from build123d import *

# Parameters (mm, degrees)
SALIENTE_EXTRUIR2_DEPTH = 3
CROQUIS2_R              = 1.25
CORTAR_EXTRUIR4_DEPTH   = 5
SALIENTE_EXTRUIR5_START = 9
CROQUIS6_R              = 2
CROQUIS6_R_2            = 1.25
SALIENTE_EXTRUIR5_DEPTH = 9
CROQUIS4_R              = 2
CROQUIS4_R_2            = 1.25
SALIENTE_EXTRUIR4_DEPTH = 5
CORTAR_EXTRUIR5_DEPTH   = 7
REDONDEO1_R             = 2


with BuildPart() as part:
    # Croquis1 → Saliente-Extruir2 (new body)
    with BuildSketch(Plane.XY):
        with BuildLine():
            Line((21.769230769, 25.846153846), (-36.230769231, 25.846153846))
            ThreePointArc((-36.230769231, 25.846153846), (-38.352089574, 24.96747419), (-39.230769231, 22.846153846))
            Line((-39.230769231, 22.846153846), (-39.230769231, -26.153846154))
            ThreePointArc((-39.230769231, -26.153846154), (-38.352089574, -28.275166497), (-36.230769231, -29.153846154))
            Line((-36.230769231, -29.153846154), (21.769230769, -29.153846154))
            ThreePointArc((21.769230769, -29.153846154), (23.890551113, -28.275166497), (24.769230769, -26.153846154))
            Line((24.769230769, -26.153846154), (24.769230769, 22.846153846))
            ThreePointArc((24.769230769, 22.846153846), (23.890551113, 24.96747419), (21.769230769, 25.846153846))
        make_face()
    extrude(amount=SALIENTE_EXTRUIR2_DEPTH)

    # Croquis2 → Cortar-Extruir4 (cut)
    with BuildSketch(Plane(origin=(0, 0, 0), x_dir=(-1, 0, 0), z_dir=(0, 0, -1))):
        with Locations((-21.769230769, 22.846153846)):
            Circle(CROQUIS2_R)
        with Locations((36.230769231, 22.846153846)):
            Circle(CROQUIS2_R)
        with Locations((36.230769231, -26.153846154)):
            Circle(CROQUIS2_R)
        with Locations((-21.769230769, -26.153846154)):
            Circle(CROQUIS2_R)
    extrude(amount=-CORTAR_EXTRUIR4_DEPTH, mode=Mode.SUBTRACT)

    # Croquis6 → Saliente-Extruir5 (add)
    # profile 1 of 4: a face of its own
    with BuildSketch(Plane(origin=(0, 0, 0), x_dir=(-1, 0, 0), z_dir=(0, 0, -1)).offset(SALIENTE_EXTRUIR5_START)):
        with Locations(Location((-21.769230769, 22.846153846, 0), (0, 0, 180))):
            Circle(CROQUIS6_R)
        with Locations((-21.769230769, 22.846153846)):
            Circle(CROQUIS6_R_2, mode=Mode.SUBTRACT)
    # profile 2 of 4: a face of its own
    with BuildSketch(Plane(origin=(0, 0, 0), x_dir=(-1, 0, 0), z_dir=(0, 0, -1)).offset(SALIENTE_EXTRUIR5_START)):
        with Locations(Location((36.230769231, 22.846153846, 0), (0, 0, 180))):
            Circle(CROQUIS6_R)
        with Locations((36.230769231, 22.846153846)):
            Circle(CROQUIS6_R_2, mode=Mode.SUBTRACT)
    # profile 3 of 4: a face of its own
    with BuildSketch(Plane(origin=(0, 0, 0), x_dir=(-1, 0, 0), z_dir=(0, 0, -1)).offset(SALIENTE_EXTRUIR5_START)):
        with Locations(Location((36.230769231, -26.153846154, 0), (0, 0, 180))):
            Circle(CROQUIS6_R)
        with Locations((36.230769231, -26.153846154)):
            Circle(CROQUIS6_R_2, mode=Mode.SUBTRACT)
    # profile 4 of 4: a face of its own
    with BuildSketch(Plane(origin=(0, 0, 0), x_dir=(-1, 0, 0), z_dir=(0, 0, -1)).offset(SALIENTE_EXTRUIR5_START)):
        with Locations(Location((-21.769230769, -26.153846154, 0), (0, 0, 180))):
            Circle(CROQUIS6_R)
        with Locations((-21.769230769, -26.153846154)):
            Circle(CROQUIS6_R_2, mode=Mode.SUBTRACT)
    extrude(amount=-SALIENTE_EXTRUIR5_DEPTH)

    # Croquis4 → Saliente-Extruir4 (add)
    # profile 1 of 3: a face of its own
    with BuildSketch(Plane.XY.offset(3)):
        with Locations((-34.230769231, -1.653846154)):
            Circle(CROQUIS4_R)
        with Locations((-34.230769231, -1.653846154)):
            Circle(CROQUIS4_R_2, mode=Mode.SUBTRACT)
    # profile 2 of 3: a face of its own
    with BuildSketch(Plane.XY.offset(3)):
        with Locations((-2.310769231, 21.746153846)):
            Circle(CROQUIS4_R)
        with Locations((-2.310769231, 21.746153846)):
            Circle(CROQUIS4_R_2, mode=Mode.SUBTRACT)
    # profile 3 of 3: a face of its own
    with BuildSketch(Plane.XY.offset(3)):
        with Locations((-2.310769231, -25.053846154)):
            Circle(CROQUIS4_R)
        with Locations((-2.310769231, -25.053846154)):
            Circle(CROQUIS4_R_2, mode=Mode.SUBTRACT)
    extrude(amount=SALIENTE_EXTRUIR4_DEPTH)

    # Croquis5 → Cortar-Extruir5 (cut)
    with BuildSketch(Plane.XY.offset(3)):
        with BuildLine():
            Line((21.769230769, 16.846153846), (-2.230769231, 16.846153846))
            Line((-2.230769231, 16.846153846), (-28.630769231, 21.10260022))
            ThreePointArc((-28.630769231, 21.10260022), (-32.183785013, 19.891309577), (-33.168405876, 16.268925289))
            Line((-33.168405876, 16.268925289), (-29.35459073, -0.548005648))
            ThreePointArc((-29.35459073, -0.548005648), (-29.230786857, -1.640569852), (-29.34878692, -2.733776112))
            Line((-29.34878692, -2.733776112), (-32.894263486, -18.761624723))
            Line((-32.894263486, -18.761624723), (-33.267463075, -20.448728388))
            ThreePointArc((-33.267463075, -20.448728388), (-31.861740508, -23.49335063), (-28.632600775, -24.398025776))
            Line((-28.632600775, -24.398025776), (-2.230769231, -20.153846154))
            Line((-2.230769231, -20.153846154), (21.769230769, -20.153846154))
            Line((21.769230769, -20.153846154), (21.769230769, 16.846153846))
        make_face()
    extrude(amount=-CORTAR_EXTRUIR5_DEPTH, mode=Mode.SUBTRACT)

    # Redondeo1
    redondeo1_edges = [part.edges().sort_by_distance(p)[0] for p in [
        (21.769230769, 16.846153846, 1.5),
        (21.769230769, -20.153846154, 1.5),
    ]]
    fillet(redondeo1_edges, radius=REDONDEO1_R)


solid = part.part
Geometry check sheet. Reference: the model listing, model coordinates, mm. A direction names the side the tool comes from. Give positions to 0.01 mm unless a question says otherwise; leave off trailing zeros. Loops run counter-clockwise (first coordinate to the right, second up) from the corner with the lowest first, then second, coordinate; pieces in that order, holes last. Notation, with made-up numbers: M -6,13.5 L 10,13.5 A21 cw 10,45.5 Z; hole C 37.5,-17 d9. An arc over 180 degrees is marked long. Write each question's results on one line, items separated by ' | '.
1) Section check C-C, the plane y = -17. Record the boundary of the cut face in (x, z).
Answers follow:
outline: M -39.23,0 L -32.5,0 L -32.5,3 L -39.23,3 Z; M 21.77,0 L 24.77,0 L 24.77,3 L 21.77,3 Z
2) Section check A-A, the plane x = 10. Record the boundary of the cut face in (y, z).
Answers follow:
outline: M -29.15,0 L -20.15,0 L -20.15,3 L -29.15,3 Z; M 16.85,0 L 25.85,0 L 25.85,3 L 16.85,3 Z
3) Section check D-D, the plane z = 1.5. Record the boundary of the cut face in (x, y), plus the area to 3 significant figures.
Answers follow:
outline: M -39.23,-26.15 A3 ccw -36.23,-29.15 L 21.77,-29.15 A3 ccw 24.77,-26.15 L 24.77,22.85 A3 ccw 21.77,25.85 L -36.23,25.85 A3 ccw -39.23,22.85 Z; hole C -36.23,-26.15 d2.5; hole C -36.23,22.85 d2.5; hole M -33.27,-20.45 A4 ccw -28.63,-24.4 L -2.23,-20.15 L 19.77,-20.15 A2 ccw 21.77,-18.15 L 21.77,14.85 A2 ccw 19.77,16.85 L -2.23,16.85 L -28.63,21.1 A4 ccw -33.17,16.27 L -29.35,-0.55 A5 cw -29.35,-2.73 Z; hole C 21.77,-26.15 d2.5; hole C 21.77,22.85 d2.5 | area: 1,390 mm2
4) Thickness scan on line 1 (Y direction, x = 19, z = 0.5); line 2 (Z direction, x = 8, y = 20); line 3 (X direction, y = 8.5, z = 1.25). Record the ranges inside material, lowest first.
Answers follow:
line 1: -29.15 to -20.15, 16.85 to 25.85 | line 2: 0 to 3 | line 3: -39.23 to -31.41, 21.77 to 24.77
5) Release check for a two-part mould opening along X. For faces 1 (the face through (-38.375, -28.252, 1.479)), 2 (the face through (23.867, -28.298, 1.479)), 3 (the face through (-12, 19, 0)) record: +X half, -X half, draft (parallel to the pull), parting line (faces both ways), or undercut.
Answers follow:
face 1: -X half | face 2: +X half | face 3: undercut
6) Gauge pin test, flat ends, axial feed: pin 1 (0.8 mm diameter, centred on x = -2, y = -25, fed in from +Z); pin 2 (1.5 mm diameter, centred on x = -2.31, y = 21.75, fed in from -Z). Record the tip position at first contact, or that the pin passes through.
Answers follow:
pin 1: z = 3 | pin 2: z = 0
7) Section check B-B, the plane z = -6.75. Record the boundary of the cut face in (x, y), plus the area to 3 significant figures.
Answers follow:
outline: C -36.23,-26.15 d4; C -36.23,22.85 d4; C 21.77,-26.15 d4; C 21.77,22.85 d4; hole C -36.23,-26.15 d2.5; hole C -36.23,22.85 d2.5; hole C 21.77,-26.15 d2.5; hole C 21.77,22.85 d2.5 | area: 30.6 mm2
8) Tool access check on faces 4 (the face through (21.17, -19.58, 1.48)), 5 (the face through (-2.57, -23.07, 5.46)), 6 (the face through (-38.33, 24.99, 1.48)), 7 (the face through (20.18, 24.06, -4.56)). Record the directions out of +Z, -Z, +X, -X, +Y, -Y that give a thin tool (end or side, any length) a straight path to the whole face; none if there is none.
Answers follow:
face 4: +Z, -Z | face 5: +Z | face 6: +Z, -Z, -X, +Y | face 7: -Z
